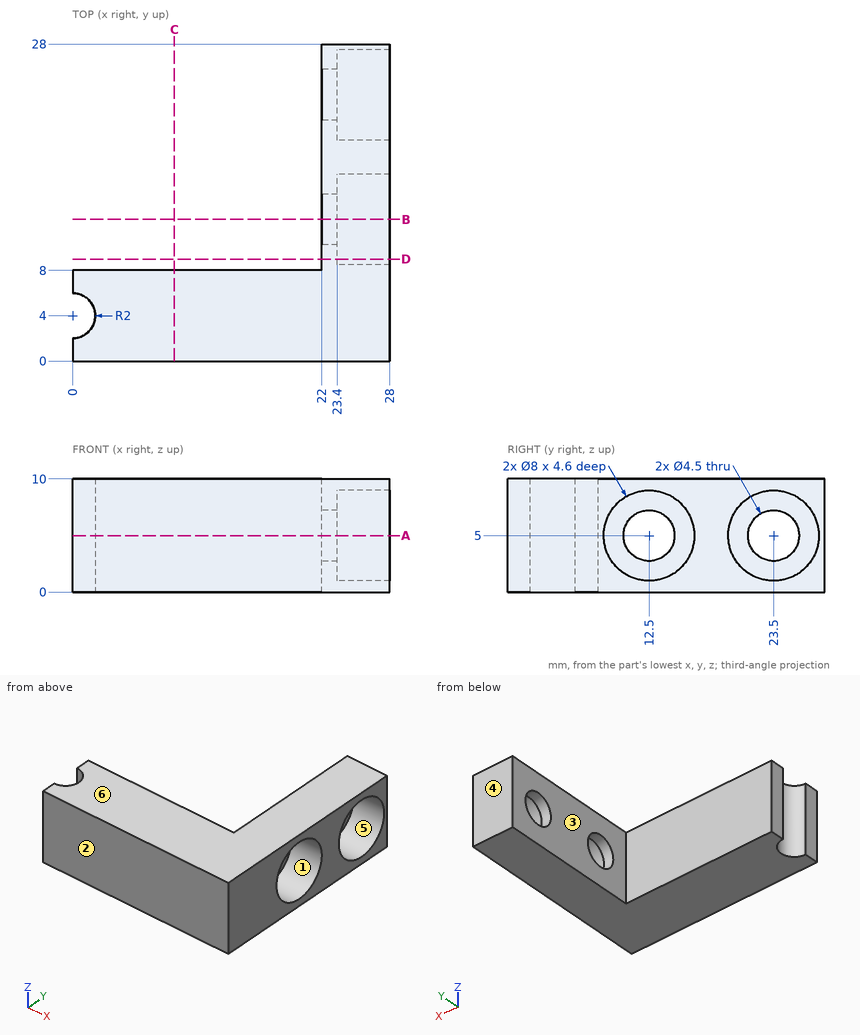
The figure shows three views and two pictorial views of one solid part (mm, origin at its lowest corner). Answer the questions. A direction names the side the tool comes from. Coordinates: 2 decimals unless noted, no trailing zeros. Loops run counter-clockwise (first coordinate to the right, second up) from the corner with the lowest first, then second, coordinate; pieces in that order, holes last. Notation, with made-up numbers: (12, -34) - (47, -34) arc R18 cw to (47, -19) - close; hole circle Ø10 at (37, 56). An arc over 180 degrees is marked (long way). Use a Markdown table: item, result. Add a question column.
1) Find the intervals of material crossed by line 1 (Y direction, x = 24.85, z = 5); line 2 (Y direction, x = 22.45, z = 5); line 3 (Z direction, x = 26.55, y = 23.5), in increasing order.
2) Given pin 1 (2 mm diameter, centred on x = 14.5, z = 2.5, fed in from +Y); pin 2 (2.5 mm diameter, centred on y = 23.5, z = 5, fed in from -X); pin 3 (2.5 mm diameter, centred on y = 23.5, z = 3.5, fed in from +X), each flat-ended and moving along its own axis, determine where each tip first touches the part or whether it passes through.
3) The part is cut by section B-B, the plane y = 12.5. Give the vertices of the cut face in (x, z).
4) The mould has two halves that part along Z. Classify the marked faces 4, 5 and 6: released by +Z, released by -Z, zero draft, split by the parting line, or undercut.
5) The part is cut by section D-D, the plane y = 9. Give the vertices of the cut face in (x, z).
6) The part is cut by section A-A, the plane z = 5. Give the vertices of the cut face in (x, y).
7) For the marked faces 1, 2 and 3, determine the directions among +Z, -Z, +X, -X, +Y, -Y from which every point of the face is accessible in a straight line to the end or side of a thin tool.
8) The part is cut by section C-C, the plane x = 9. Give the vertices of the cut face in (y, z), and give its area (3 significant figures).
Here are the results:
| question | item | result |
|---|---|---|
| 1 | line 1 | y = 0 to 8.5, 16.5 to 19.5, 27.5 to 28 |
| 1 | line 2 | y = 0 to 10.25, 14.75 to 21.25, 25.75 to 28 |
| 1 | line 3 | z = 0 to 1, 9 to 10 |
| 2 | pin 1 | stops at y = 8 |
| 2 | pin 2 | passes through |
| 2 | pin 3 | stops at x = 23.4 |
| 3 | outline | (22, 0) - (28, 0) - (28, 1) - (23.4, 1) - (23.4, 2.75) - (22, 2.75) - close; (22, 7.25) - (23.4, 7.25) - (23.4, 9) - (28, 9) - (28, 10) - (22, 10) - close |
| 4 | face 4 | zero draft |
| 4 | face 5 | undercut |
| 4 | face 6 | released by +Z |
| 5 | outline | (22, 0) - (28, 0) - (28, 3.06) - (23.4, 3.06) - (23.4, 6.94) - (28, 6.94) - (28, 10) - (22, 10) - close |
| 6 | outline | (0, 0) - (28, 0) - (28, 8.5) - (23.4, 8.5) - (23.4, 10.25) - (22, 10.25) - (22, 8) - (0, 8) - (0, 6) arc R2 cw to (0, 2) - close; (22, 14.75) - (23.4, 14.75) - (23.4, 16.5) - (28, 16.5) - (28, 19.5) - (23.4, 19.5) - (23.4, 21.25) - (22, 21.25) - close; (22, 25.75) - (23.4, 25.75) - (23.4, 27.5) - (28, 27.5) - (28, 28) - (22, 28) - close |
| 7 | face 1 | +X |
| 7 | face 2 | +Z, -Z, +X, -X, -Y |
| 7 | face 3 | +Z, -Z, -X, +Y |
| 8 | outline | (0, 0) - (8, 0) - (8, 10) - (0, 10) - close |
| 8 | area | 80.0 mm^2 |
